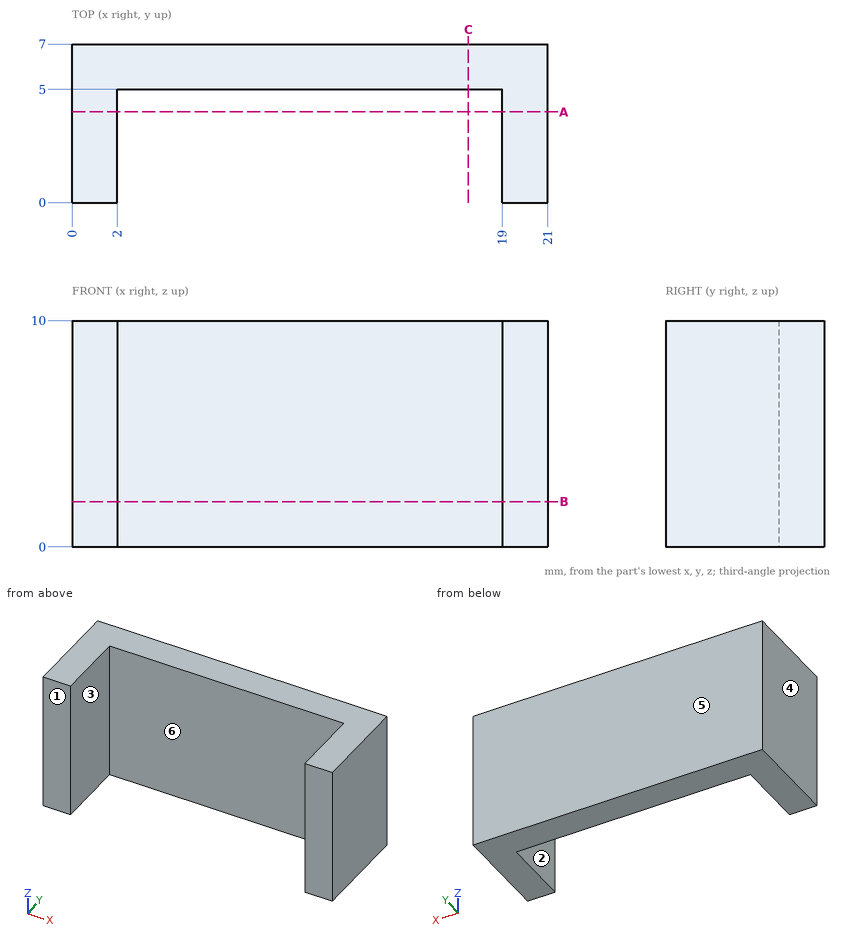
Geometry: see drawing. Coordinates: mm, zero at the bounding-box minimum. A direction names the side the tool comes from. Round coordinates to 2 decimals unless told otherwise and drop trailing zeros. Write each loop counter-clockwise with the first axis right and the second up, starting at its lowest first coordinate (ties: lowest second). Pieces come first, ordered by that corner, then holes.
1) Contact query for a flat-ended pin moving along its axis: P1, Ø1, axis at x = 17.5, y = 4, coming from the -Z side. Output: stop coordinate, or through.
2) Cut plane A-A (y = 4). Return the cut outline in (x, z).
3) Ray query, L1, parallel to X at y = 1.5, z = 3; L2, parallel to Y at x = 11.25, z = 8.5. Return the intervals inside material, ascending.
4) Draft query along X for the marked faces 3, 4, 5 and 6. Return one class per face: pulls with the +X half, pulls with the -X half, needs draft (parallel to the pull), parting line crosses it, or undercut.
5) Cut plane B-B (z = 2). Return the cut outline in (x, y).
6) Cut plane C-C (x = 17.5). Return the cut outline in (y, z), then the cut area to 3 significant figures.
7) Reachability of the marked faces 1 and 2 from +Z, -Z, +X, -X, +Y, -Y: full face, straight path, thin tool, end or side. Return the list, or none.
Geometry says:
1. P1: passes through
2. outline: (0, 0) - (2, 0) - (2, 10) - (0, 10) - close; (19, 0) - (21, 0) - (21, 10) - (19, 10) - close
3. L1: x = 0 to 2, 19 to 21
3. L2: y = 5 to 7
4. face 3: undercut
4. face 4: pulls with the -X half
4. face 5: needs draft
4. face 6: undercut
5. outline: (0, 0) - (2, 0) - (2, 5) - (19, 5) - (19, 0) - (21, 0) - (21, 7) - (0, 7) - close
6. outline: (5, 0) - (7, 0) - (7, 10) - (5, 10) - close
6. area: 20.0 mm2
7. face 1: +Z, -Z, +X, -X, -Y
7. face 2: +Z, -Z, -Y
